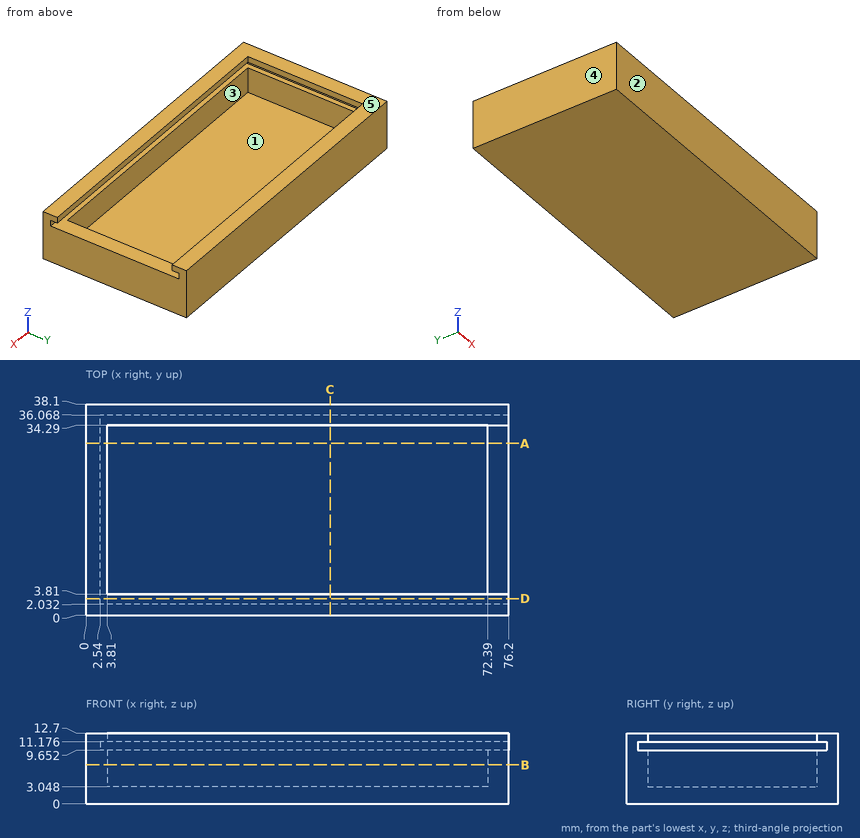
Source: three-view drawing plus pictorial views. Frame: mm from the lowest corner of the part. A direction names the side the tool comes from. Round coordinates to 2 decimals unless told otherwise and drop trailing zeros. Loops run counter-clockwise (first coordinate to the right, second up) from the corner with the lowest first, then second, coordinate; pieces in that order, holes last. Notation, with made-up numbers: M 63.5,73.5 L 97.5,73.5 A21 ccw 97.5,78.5 Z; hole C 24.5,-7.5 d10. An arc over 180 degrees is marked long. Answer as CSV lines item,"result".
Q1. Pull-direction query (X, two-part tool) for the marked faces 3, 4 and 5; classes: +X half, -X half, draft (parallel to the pull), parting line (faces both ways), or undercut.
Verdict:
face 3,"undercut"
face 4,"-X half"
face 5,"draft"
Q2. Line query: line 1 along Y through (x, z) = (34, 12); line 2 along Y through (x, z) = (56, 10.5); line 3 along X through (y, z) = (21.5, 6.5). Output: solid intervals per line, ascending.
Verdict:
line 1,"y = 0 to 3.81, 34.29 to 38.1"
line 2,"y = 0 to 2.03, 36.07 to 38.1"
line 3,"x = 0 to 3.81, 72.39 to 76.2"
Q3. Cut plane A-A (y = 31). Return the cut outline in (x, z).
Verdict:
outline,"M 0,0 L 76.2,0 L 76.2,9.65 L 72.39,9.65 L 72.39,3.05 L 3.81,3.05 L 3.81,9.65 L 2.54,9.65 L 2.54,11.18 L 3.81,11.18 L 3.81,12.7 L 0,12.7 Z"
Q4. Cut plane C-C (x = 44). Return the cut outline in (y, z).
Verdict:
outline,"M 0,0 L 38.1,0 L 38.1,12.7 L 34.29,12.7 L 34.29,11.18 L 36.07,11.18 L 36.07,9.65 L 34.29,9.65 L 34.29,3.05 L 3.81,3.05 L 3.81,9.65 L 2.03,9.65 L 2.03,11.18 L 3.81,11.18 L 3.81,12.7 L 0,12.7 Z"
Q5. Cut plane D-D (y = 3). Return the cut outline in (x, z).
Verdict:
outline,"M 0,0 L 76.2,0 L 76.2,9.65 L 2.54,9.65 L 2.54,11.18 L 76.2,11.18 L 76.2,12.7 L 0,12.7 Z"
Q6. Reachability of the marked faces 1 and 2 from +Z, -Z, +X, -X, +Y, -Y: full face, straight path, thin tool, end or side. Return the list, or none.
Verdict:
face 1,"+Z"
face 2,"+Z, -Z, +X, -X, -Y"
Q7. Cut plane B-B (z = 7). Return the cut outline in (x, y), plus the area to 3 significant figures.
Verdict:
outline,"M 0,0 L 76.2,0 L 76.2,38.1 L 0,38.1 Z; hole M 3.81,3.81 L 72.39,3.81 L 72.39,34.29 L 3.81,34.29 Z"
area,"813 mm^2"
Q8. Contact query for flat-ended pins moving along their axis: pin 1 (12 mm diameter, centred on x = 44, y = 15.5, fed in from +Z); pin 2 (1.2 mm diameter, centred on y = 13, z = 10.5, fed in from +X); pin 3 (0.8 mm diameter, centred on y = 21.5, z = 12, fed in from +X). Output: stop coordinate, or through.
Verdict:
pin 1,"stops at z = 3.05"
pin 2,"stops at x = 2.54"
pin 3,"stops at x = 3.81"
